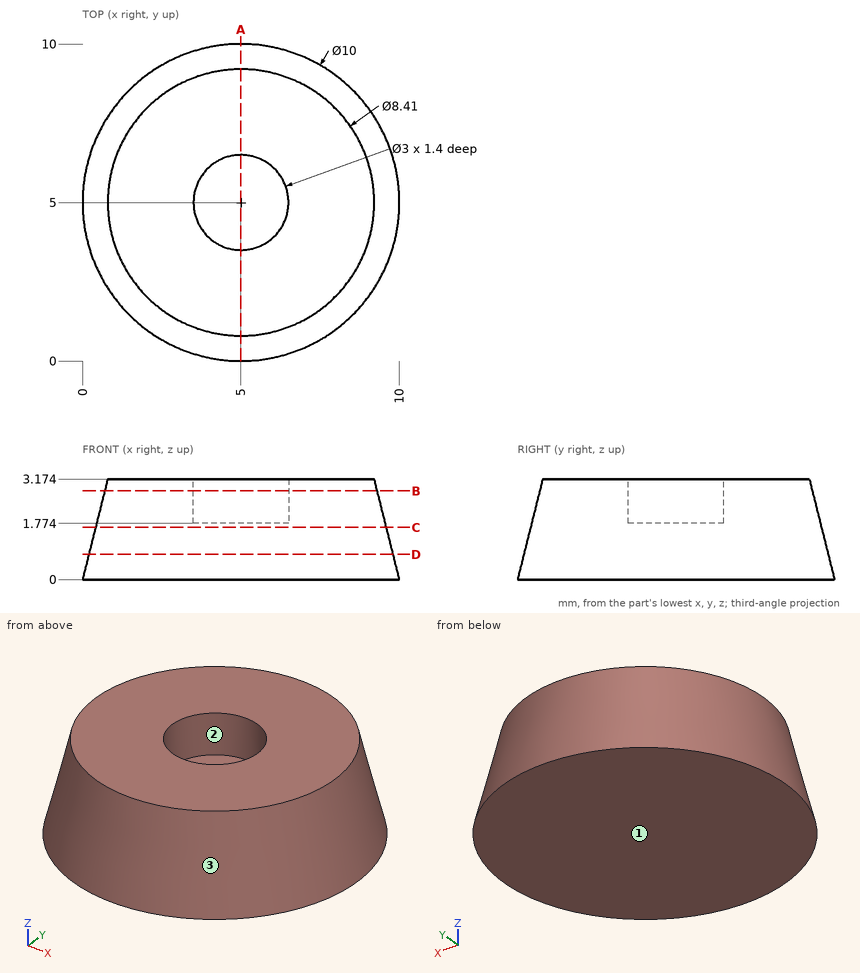
Design review of the part shown in the three views and the two pictorial views. Dimensions are in mm from the part's minimum x, y and z. Coordinates: 2 decimals unless noted, no trailing zeros. Order: outer loops, then holes, each group sorted by start corner. A loop starts at its lowest first (then second) coordinate and runs counter-clockwise, first axis right, second up.
Item 1: The part is to be moulded in two halves that separate along Y. For the marked faces 1, 2 and 3, say which applies: pulls with the +Y half, pulls with the -Y half, needs draft (parallel to the pull), parting line crosses it, or undercut.
Item 2: Take a section at A-A, the plane x = 5. Write out the cut boundary in (y, z) (3 decimals), then the cut area to 3 significant figures.
Item 3: Take a section at D-D, the plane z = 0.8. Write out the cut boundary in (x, y).
Item 4: Take a section at B-B, the plane z = 2.8. Write out the cut boundary in (x, y).
Item 5: For line 1 (Z direction, x = 4, y = 4.5); line 2 (X direction, y = 4.75, z = 1.9); line 3 (Y direction, x = 5, z = 2.85), list the stretches that pass through material, from the lowest coordinate up.
Item 6: Take a section at C-C, the plane z = 1.65. Write out the cut boundary in (x, y).
Item 7: For pin 1 Ø0.9 at (x, y) = (5.5, 5.5) entering from +Z, flat-tipped, find the tip position at first contact; note if it passes through.
The answers:
1. face 1: needs draft
1. face 2: undercut
1. face 3: parting line crosses it
2. outline: (0, 0) - (10, 0) - (9.205, 3.174) - (6.5, 3.174) - (6.5, 1.774) - (3.5, 1.774) - (3.5, 3.174) - (0.795, 3.174) - close
2. area: 25.0 mm2
3. outline: circle Ø9.6 at (5, 5)
4. outline: circle Ø8.6 at (5, 5); hole circle Ø3 at (5, 5)
5. line 1: z = 0 to 1.77
5. line 2: x = 0.48 to 3.52, 6.48 to 9.52
5. line 3: y = 0.71 to 3.5, 6.5 to 9.29
6. outline: circle Ø9.17 at (5, 5)
7. pin 1: stops at z = 1.77
